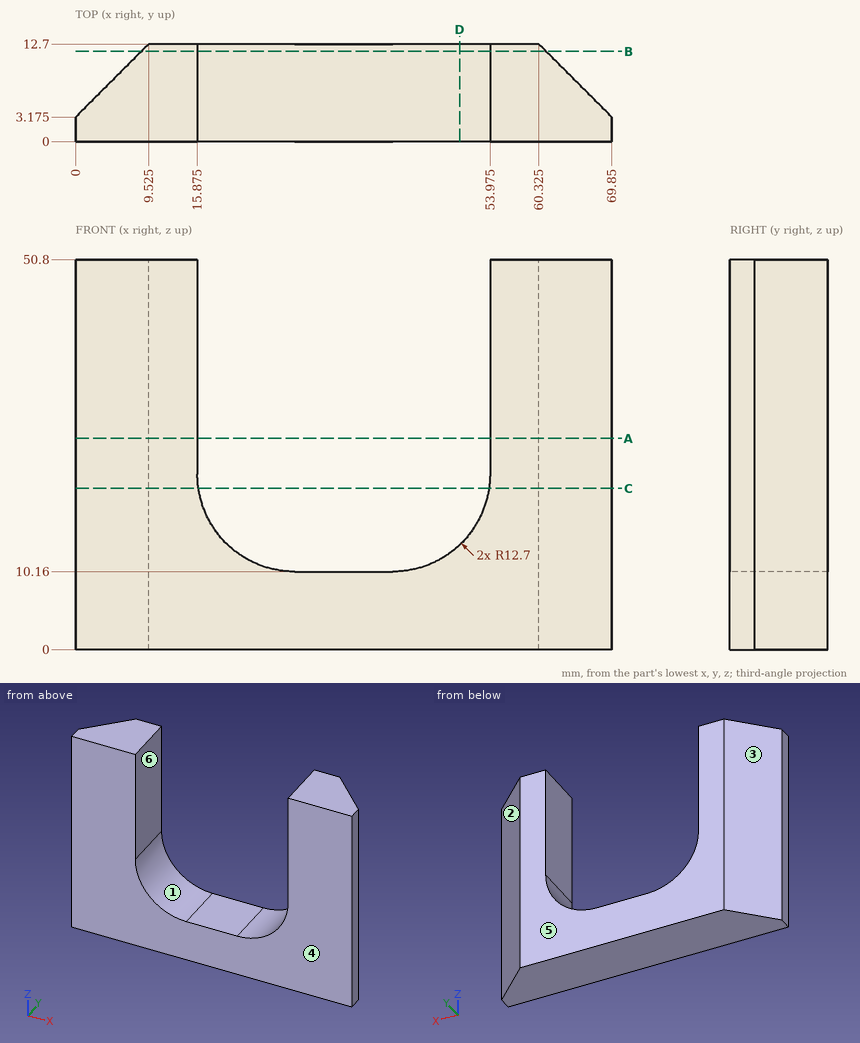
Answer from the drawing. Dimensions are ordinates in mm from the lowest x, y and z of the part. A direction names the side the tool comes from. Coordinates: 2 decimals unless noted, no trailing zeros. Write each loop counter-clockwise with the first axis right and the second up, starting at its lowest first coordinate (ties: lowest second). Pieces come first, ordered by that corner, then holes. Notation, with made-up numbers: (-18, 27) - (38, 27) arc R21 cw to (38, 41) - close; hole circle Ø2 at (29, 75.5). An arc over 180 degrees is marked (long way). Return JSON: item names as keys, results as strings. Group by question number.
Q1. The part is cut by section C-C on z = 21. Write down the section's boundary in (x, y) (3 decimals).
Q2. Which of the six approach directions +Z, -Z, +X, -X, +Y, -Y give full straight-line access (tool end or side, diameter ignored) to the marked faces 5 and 6?
Q3. The part is cut by section B-B on y = 11.75. Write down the section's boundary in (x, z) (3 decimals).
Q4. The part is cut by section A-A on z = 27.5. Write down the section's boundary in (x, y) (3 decimals), and give its area (4 significant figures).
Q5. Flat-ended cylindrical pins translate along their axes: pin 1 Ø3 at (y, z) = (7, 11) entering from -X (3 decimals); pin 2 Ø4 at (y, z) = (6.5, 21.5) entering from +X (3 decimals); pin 3 Ø10 at (x, z) = (28.5, 19.5) entering from +Y. Find the tip coordinate at first contact, or state that the pin passes through.
Q6. For a pull along X with two mould halves and no side action, classify the marked faces 1, 2, 3 and 4 as +X half, -X half, draft (parallel to the pull), parting line (faces both ways), or undercut.
Q7. Find the intervals of material crossed by line 1 along Z through (x, y) = (31, 2.75); line 2 along X through (y, z) = (3.75, 36.5) (3 decimals); line 3 along X through (y, z) = (3, 28) (3 decimals), in increasing order. Write a range as [from, to].
Q8. The part is cut by section D-D on x = 50. Write down the section's boundary in (y, z), and give its area (3 significant figures).
Evaluation:
{
 "1": {"outline": "(0, 0) - (16.012, 0) - (16.012, 12.7) - (9.525, 12.7) - (0, 3.175) - close; (53.838, 0) - (69.85, 0) - (69.85, 3.175) - (60.325, 12.7) - (53.838, 12.7) - close"},
 "2": {"face 5": "+Z, -Z, +X, -X, +Y", "face 6": "+Z, +Y, -Y"},
 "3": {"outline": "(8.575, 0) - (61.275, 0) - (61.275, 50.8) - (53.975, 50.8) - (53.975, 22.86) arc R12.7 cw to (41.275, 10.16) - (28.575, 10.16) arc R12.7 cw to (15.875, 22.86) - (15.875, 50.8) - (8.575, 50.8) - close"},
 "4": {"outline": "(0, 0) - (15.875, 0) - (15.875, 12.7) - (9.525, 12.7) - (0, 3.175) - close; (53.975, 0) - (69.85, 0) - (69.85, 3.175) - (60.325, 12.7) - (53.975, 12.7) - close", "area": "312.5 mm2"},
 "5": {"pin 1": "stops at x = 2.325", "pin 2": "stops at x = 68.525", "pin 3": "passes through"},
 "6": {"face 1": "undercut", "face 2": "+X half", "face 3": "-X half", "face 4": "draft"},
 "7": {"line 1": "z = [0, 10.16]", "line 2": "x = [0.575, 15.875], [53.975, 69.275]", "line 3": "x = [0, 15.875], [53.975, 69.85]"},
 "8": {"outline": "(0, 0) - (12.7, 0) - (12.7, 13.63) - (0, 13.63) - close", "area": "173 mm2"}
}
